```python
from build123d import *

# Parameters (mm, degrees)
F1_DEPTH    = 20
F2_R        = 1.8
F3_DEPTH    = 30.001
F4_SIZE2    = 14
F4_SIZE     = 26
F5_SIZE     = 2
F6_R        = 4
F7_T1_DEPTH = 13.9458816311
F7_T3_DEPTH = 13.9458816311
F8_W        = 2
F8_H        = 5
F9_DEPTH    = 30.001
F10_SIZE    = 1.99999


# Not quite as in the source:
# - a fillet or chamfer that OpenCascade refuses, or shapes differently, is made with other operations: its cross-section is extruded or revolved along the edge and cut away or added
# - a fillet or chamfer is up to 0.001 mm smaller than in the source, because OpenCascade refuses the exact size


with BuildPart() as f1:
    # F0 (on Top) → F1 (new body)
    with BuildSketch(Plane.XY):
        Polygon((15, 13), (13, 13), (13, -13), (-13, -13), (-13, 13), (-15, 13), (-15, -17), (15, -17), align=None)
    extrude(amount=F1_DEPTH)

    # F2 (on face) → F3 (cut, through all)
    with BuildSketch(Plane.YZ.offset(15)):
        with Locations((9.7, 3.3)):
            Circle(F2_R)
    extrude(amount=-F3_DEPTH, mode=Mode.SUBTRACT)

    # F4
    f4_edges = [f1.edges().sort_by_distance(p)[0] for p in [
        (14, 13, 20),
        (-14, 13, 20),
    ]]
    f4_side = f1.faces().sort_by_distance((14, 12.575736, 20))[0]
    chamfer(f4_edges, length=F4_SIZE, length2=F4_SIZE2, reference=f4_side)

    # F5
    f5_edges = [f1.edges().sort_by_distance(p)[0] for p in [
        (14, 13, 0),
        (-14, 13, 0),
    ]]
    chamfer(f5_edges, length=F5_SIZE)

    # F6
    f6_edges = [f1.edges().sort_by_distance(p)[0] for p in [
        (14, 13, 2),
        (-14, 13, 2),
    ]]
    fillet(f6_edges, radius=F6_R)

    # F7: fillet of radius 4 on 2 edges, made by hand

    # F7_s2 → F7_t1 (cut)
    with BuildSketch(Plane.YZ.offset(7.0270591844)):
        with BuildLine():
            ThreePointArc((13, 3.6108236738), (12.4340644409, 5.66197004), (10.8963992921, 7.1327080735))
            Line((10.8963992921, 7.1327080735), (13, 6))
            Line((13, 6), (13, 3.6108236738))
        make_face()
    extrude(amount=F7_T1_DEPTH, mode=Mode.SUBTRACT)

    # F7_s4 → F7_t3 (cut)
    with BuildSketch(Plane.YZ.offset(-20.9729408156)):
        with BuildLine():
            ThreePointArc((10.8963992921, 7.1327080735), (12.4340644409, 5.66197004), (13, 3.6108236738))
            Line((13, 3.6108236738), (13, 6))
            Line((13, 6), (10.8963992921, 7.1327080735))
        make_face()
    extrude(amount=F7_T3_DEPTH, mode=Mode.SUBTRACT)

    # F8 (on face) → F9 (cut, through all)
    with BuildSketch(Plane.YZ.offset(15)):
        with Locations((-14, 14.5)):
            Rectangle(F8_W, F8_H)
        with Locations((-14, 5.5)):
            Rectangle(F8_W, F8_H)
    extrude(amount=-F9_DEPTH, mode=Mode.SUBTRACT)

    # F10 (size 2 in the source; OpenCascade refuses exactly that, so slightly less here)
    f10_edges = [f1.edges().sort_by_distance(p)[0] for p in [
        (0, -13, 8),
        (0, -13, 17),
    ]]
    chamfer(f10_edges, length=F10_SIZE)


solid = f1.part
```
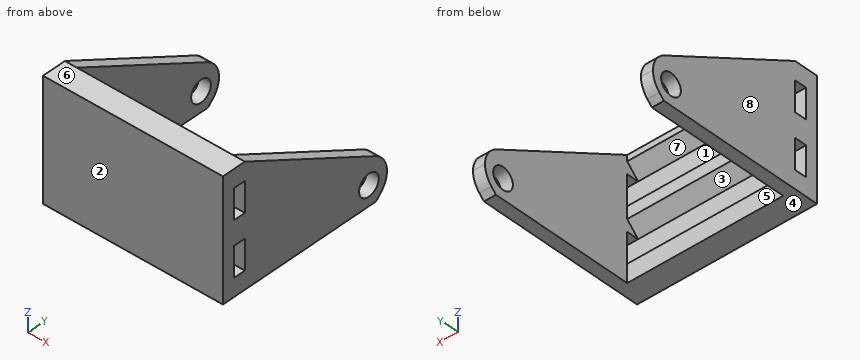
Verification items for the finished model (mm, model axes). Face numbers are marked on the shaded views. A direction names the side the tool comes from. Give positions to 0.01 mm unless a question says otherwise; leave off trailing zeros. Write each loop counter-clockwise with the first axis right and the second up, starting at its lowest first coordinate (ties: lowest second). Pieces come first, ordered by that corner, then holes. Notation, with made-up numbers: M -23.5,-34.5 L -13.5,-34.5 A11 cw -13.5,-26.5 Z; hole C 49,-34.75 d11. An arc over 180 degrees is marked long. One line per question, with ' | ' between items.
1) Section check A-A on y = -11.5. Enter the section's corners in (x, z), plus the area to 3 significant figures.
Result:
outline: M -15,0 L -13,0 L -13,19.19 L -15,19.19 Z; M 13,0 L 15,0 L 15,19.19 L 13,19.19 Z | area: 76.8 mm2
2) Section check B-B on z = 11.25. Enter the section's corners in (x, y), plus the area to 3 significant figures.
Result:
outline: M -15,-17 L 15,-17 L 15,3.25 L 13,3.25 L 13,-13 L -13,-13 L -13,3.25 L -15,3.25 Z | area: 185 mm2
3) Set-up check for the marked faces 1, 2, 3, 4 and 5: record each of +Z, -Z, +X, -X, +Y, -Y from which the full face is reachable in a straight line by a thin tool's end or side.
Result:
face 1: +X, -X | face 2: +Z, -Z, +X, -X, -Y | face 3: +Y | face 4: -Z, +X, -X, +Y, -Y | face 5: +Z, -Z, +Y
4) Mould release check, pull along X, two halves, no side actions. Record for the marked faces 6, 7 and 8: released by +X, released by -X, zero draft, split by the parting line, or undercut.
Result:
face 6: zero draft | face 7: undercut | face 8: released by -X
5) Section check D-D on y = 9.7. Enter the section's corners in (x, z), plus the area to 3 significant figures.
Result:
outline: M -15,0 L -13,0 L -13,1.5 L -15,1.5 Z; M -15,5.1 L -13,5.1 L -13,7.78 L -15,7.78 Z; M 13,0 L 15,0 L 15,1.5 L 13,1.5 Z; M 13,5.1 L 15,5.1 L 15,7.78 L 13,7.78 Z | area: 16.7 mm2
6) Gauge pin test, flat ends, axial feed: pin 1 Ø4 at (x, z) = (-4, 6.5) entering from +Y; pin 2 Ø2 at (y, z) = (2.5, 13.5) entering from -X; pin 3 Ø1.5 at (x, z) = (5, 1.5) entering from +Y. Record the tip position at first contact, or that the pin passes through.
Result:
pin 1: stops at y = -14.5 | pin 2: passes through | pin 3: stops at y = -13
7) Thickness scan on line 1 along X through (y, z) = (-4.75, 12); line 2 along Y through (x, z) = (-3.5, 13); line 3 along Z through (x, y) = (14.65, 9.7). Record the ranges inside material, lowest first. Write a range as [from, to].
Result:
line 1: x = [-15, -13], [13, 15] | line 2: y = [-17, -15] | line 3: z = [0, 1.5], [5.1, 7.78]
